```python
from build123d import *

# Parameters (mm, degrees)
F0_W     = 65.630324
F0_H     = 62.311936
F1_DEPTH = 25.4
F2_R     = 8.207931
F3_DEPTH = 25.401
F4_W     = 15.485808
F4_H     = 18.435483
F5_DEPTH = 25.4


with BuildPart() as f1:
    # F0 (on Front) → F1 (new body)
    with BuildSketch(Plane.XZ):
        Rectangle(F0_W, F0_H)
    extrude(amount=F1_DEPTH)

    # F2 (on face) → F3 (cut, through all)
    with BuildSketch(Plane.XZ.offset(25.4)):
        with Locations((-14.278099, 16.009722)):
            Circle(F2_R)
    extrude(amount=-F3_DEPTH, mode=Mode.SUBTRACT)

    # F4 (on face) → F5 (cut)
    with BuildSketch(Plane.XZ.offset(25.4)):
        with Locations((6.268065, -18.251129)):
            Rectangle(F4_W, F4_H)
    extrude(amount=-F5_DEPTH, mode=Mode.SUBTRACT)


solid = f1.part
```
For this review, take the finished solid that the model builds, in its own axes (mm). A direction names the side the tool comes from. Give positions to 0.01 mm unless a question says otherwise; leave off trailing zeros. Order: outer loops, then holes, each group sorted by start corner. A loop starts at its lowest first (then second) coordinate and runs counter-clockwise, first axis right, second up.
1) Wall thickness on line 1 (Z direction, x = 6, y = -20.5); line 2 (X direction, y = -16.5, z = -9.5); line 3 (Z direction, x = -9.5, y = -1): over which ranges is each line inside the solid? List them lowest first.
2) Take a section at A-A (x = 6). Give the boundary of the cut face in (y, z).
3) Insertion check: pin 1 (2 mm diameter, centred on x = -3.5, z = 4, fed in from +Y). The pin has a flat end and moves straight along its axis. Give the tip position at first contact, or say it passes through.
4) For faces 5 (the face through (0, -25.4, 0)), 6 (the face through (6, -13, -9.033)), list the 3-axis set-ups (+Z, -Z, +X, -X, +Y, -Y) from which the entire face can be reached by the end or side of a thin tool; tool diameter is ignored.
5) The part is to be moulded in two halves that separate along X. For faces 1 (the face through (0, -13, -31.156)), 2 (the face through (-1.475, -13, -18)), 3 (the face through (14.011, -13, -18)), 4 (the face through (-32.815, -13, 0)), say which applies: released by +X, released by -X, zero draft, split by the parting line, or undercut.
6) Take a section at C-C (y = -5.5). Give the boundary of the cut face in (x, z), then the cut area to 3 significant figures.
7) Take a section at B-B (z = -11). Give the boundary of the cut face in (x, y).
Derived:
1. line 1: z = -31.16 to -27.47, -9.03 to 31.16
1. line 2: x = -32.82 to -1.47, 14.01 to 32.82
1. line 3: z = -31.16 to 9.34, 22.68 to 31.16
2. outline: (-25.4, -31.16) - (0, -31.16) - (0, -27.47) - (-25.4, -27.47) - close; (-25.4, -9.03) - (0, -9.03) - (0, 31.16) - (-25.4, 31.16) - close
3. pin 1: stops at y = 0
4. face 5: +Z, -Z, +X, -X, -Y
4. face 6: +Y, -Y
5. face 1: zero draft
5. face 2: undercut
5. face 3: undercut
5. face 4: released by -X
6. outline: (-32.82, -31.16) - (32.82, -31.16) - (32.82, 31.16) - (-32.82, 31.16) - close; hole circle Ø16.42 at (-14.28, 16.01); hole (-1.47, -27.47) - (14.01, -27.47) - (14.01, -9.03) - (-1.47, -9.03) - close
6. area: 3,590 mm2
7. outline: (-32.82, -25.4) - (-1.47, -25.4) - (-1.47, 0) - (-32.82, 0) - close; (14.01, -25.4) - (32.82, -25.4) - (32.82, 0) - (14.01, 0) - close
